from build123d import *

# Parameters (mm, degrees)
EXTRUDE_1_DEPTH          = 20
FILLET_1_R               = 3
CUT_EXTRUDE_1_DEPTH      = 75.37216767
CUT_EXTRUDE_1_DEPTH_BACK = 75.37216767
SKETCH_2_R               = 2.7
SKETCH_2_R_2             = 2.3


with BuildPart() as part:
    # 草图1 → 凸台-拉伸1 (new body)
    with BuildSketch(Plane.XY):
        with BuildLine():
            Line((54.2, 3.8), (54.2, 0.3))
            Line((54.2, 0.3), (70.972736483, 0.3))
            Line((70.972736483, 0.3), (70.972736483, 3.3))
            Line((70.972736483, 3.3), (64.032462364, 3.3))
            ThreePointArc((64.032462364, 3.3), (60.620717942, 4.364414928), (58.419477418, 7.18))
            ThreePointArc((58.419477418, 7.18), (50, 13), (41.580522582, 7.18))
            ThreePointArc((41.580522582, 7.18), (39.379282058, 4.364414928), (35.967537636, 3.3))
            Line((35.967537636, 3.3), (-35.967537636, 3.3))
            ThreePointArc((-35.967537636, 3.3), (-39.379282058, 4.364414928), (-41.580522582, 7.18))
            ThreePointArc((-41.580522582, 7.18), (-50, 13), (-58.419477418, 7.18))
            ThreePointArc((-58.419477418, 7.18), (-60.620717942, 4.364414928), (-64.032462364, 3.3))
            Line((-64.032462364, 3.3), (-70.972736483, 3.3))
            Line((-70.972736483, 3.3), (-70.972736483, 0.3))
            Line((-70.972736483, 0.3), (-54.2, 0.3))
            Line((-54.2, 0.3), (-54.2, 3.8))
            ThreePointArc((-54.2, 3.8), (-50, 8), (-45.8, 3.8))
            Line((-45.8, 3.8), (-45.8, 0.3))
            Line((-45.8, 0.3), (45.8, 0.3))
            Line((45.8, 0.3), (45.8, 3.8))
            ThreePointArc((45.8, 3.8), (50, 8), (54.2, 3.8))
        make_face()
    extrude(amount=EXTRUDE_1_DEPTH)

    # 圆角1
    fillet_1_edges = [part.edges().sort_by_distance(p)[0] for p in [
        (70.972736483, 1.8, 20),
        (-70.972736483, 1.8, 0),
        (70.972736483, 1.8, 0),
        (-70.972736483, 1.8, 20),
    ]]
    fillet(fillet_1_edges, radius=FILLET_1_R)

    # 草图2 → 切除-拉伸1 (cut, two sides: drawn at the far end of the back side and taken through both)
    with BuildSketch(Plane(origin=(0, 3.3, 0), x_dir=(1, 0, 0), z_dir=(0, 1, 0)).offset(-CUT_EXTRUDE_1_DEPTH_BACK)):
        with Locations(Location((0, -10, 0), (0, 0, 270))):
            Circle(SKETCH_2_R)
        with Locations(Location((66.372736483, -10, 0), (0, 0, 270))):
            Circle(SKETCH_2_R_2)
        with Locations(Location((33.627263517, -10, 0), (0, 0, 270))):
            Circle(SKETCH_2_R_2)
        with Locations(Location((-33.627263517, -10, 0), (0, 0, 270))):
            Circle(SKETCH_2_R_2)
        with Locations(Location((-66.372736483, -10, 0), (0, 0, 270))):
            Circle(SKETCH_2_R_2)
    extrude(amount=CUT_EXTRUDE_1_DEPTH + CUT_EXTRUDE_1_DEPTH_BACK, mode=Mode.SUBTRACT)


solid = part.part
Verification items for the finished model (mm, model axes). A direction names the side the tool comes from. Round coordinates to 2 decimals unless told otherwise and drop trailing zeros. Write each loop counter-clockwise with the first axis right and the second up, starting at its lowest first coordinate (ties: lowest second). Pieces come first, ordered by that corner, then holes.
(1) Depth check by flat-ended pin: pin 1 Ø3 at (x, z) = (-29.5, 7.5) entering from +Y; pin 2 Ø3.5 at (x, z) = (33.63, 10) entering from +Y; pin 3 Ø1 at (y, z) = (7, 2.5) entering from +X. Enter the tip coordinate at first touch or a pass-through.
Returned:
pin 1: stops at y = 3.3
pin 2: passes through
pin 3: stops at x = 58.73
(2) Section check A-A (x = 0). Enter the section's corners in (y, z), plus the area to 3 significant figures.
Returned:
outline: (0.3, 0) - (3.3, 0) - (3.3, 7.3) - (0.3, 7.3) - close; (0.3, 12.7) - (3.3, 12.7) - (3.3, 20) - (0.3, 20) - close
area: 43.8 mm2
(3) Section check D-D (x = 15). Enter the section's corners in (y, z), plus the area to 3 significant figures.
Returned:
outline: (0.3, 0) - (3.3, 0) - (3.3, 20) - (0.3, 20) - close
area: 60.0 mm2
(4) Material ranges on line 1 (Z direction, x = 0, y = 2.65); line 2 (X direction, y = 7.5, z = 4); line 3 (X direction, y = 6.75, z = 5), recorded low to high.
Returned:
line 1: z = 0 to 7.3, 12.7 to 20
line 2: x = -58.29 to -51.99, -48.01 to -41.71, 41.71 to 48.01, 51.99 to 58.29
line 3: x = -58.6 to -52.99, -47.01 to -41.4, 41.4 to 47.01, 52.99 to 58.6
(5) Mould release check, pull along Z, two halves, no side actions. Record for faces 5 (the cylindrical face through (-70.117, 1.779, 19.098)), 6 (the cylindrical face through (-50, 13, 10)), 7 (the cylindrical face through (35.908, 1.779, 9.701)): pulls with the +Z half, pulls with the -Z half, needs draft (parallel to the pull), parting line crosses it, or undercut.
Returned:
face 5: pulls with the +Z half
face 6: needs draft
face 7: undercut
(6) Section check B-B (z = 10). Give the number of separate pieces and of enclosed holes in the cut face, plus the area to 3 significant figures.
Returned:
separate pieces: 6
enclosed holes: 0
area: 537 mm2
(7) Section check C-C (x = 50). Enter the section's corners in (y, z).
Returned:
outline: (8, 0) - (13, 0) - (13, 20) - (8, 20) - close
(8) Access from +Z, -Z, +X, -X, +Y, -Y to the whole of each face (thin tool, end or side, straight path). Record for faces 1 (the flat face through (-45.8, 2, 10)), 2 (the cylindrical face through (70.117, 1.821, 0.902)), 3 (the cylindrical face through (39.421, 4.393, 9.86)), 4 (the flat face through (-69, 3.3, 10)).
Returned:
face 1: +Z, -Z, -Y
face 2: -Z, +X, +Y, -Y
face 3: +Z, -Z, +Y
face 4: +Z, -Z, -X, +Y
